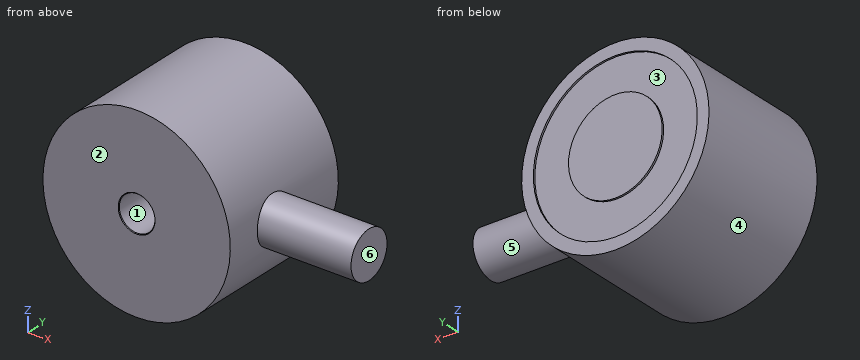
```python
from build123d import *

# Parameters (mm, degrees)
SKETCH1_R           = 12.7
BOSS_EXTRUDE1_DEPTH = 19.05
SKETCH2_W           = 4.7625
SKETCH2_H           = 0.254
SKETCH3_R           = 2.413
CUT_EXTRUDE1_DEPTH  = 9.525
BOSS_EXTRUDE2_START = 25.4
SKETCH7_R           = 3.175
BOSS_EXTRUDE2_DEPTH = 13.103277876


# Read off the part's stored shape, not the designer's step: Cut-Extrude2
with BuildPart() as part:
    # Sketch1 → Boss-Extrude1 (new body)
    with BuildSketch(Plane(origin=(0, 0, 0), x_dir=(1, 0, 0), z_dir=(0, 1, 0))):
        with Locations(Location((0, 0, 0), (0, 0, 90))):
            Circle(SKETCH1_R)
    extrude(amount=BOSS_EXTRUDE1_DEPTH)

    # Sketch2 → Cut-Revolve1 (revolve, cut)
    with BuildSketch(Plane.XY, mode=Mode.PRIVATE) as cut_revolve1_sk:
        with Locations((-8.73125, 18.923)):
            Rectangle(SKETCH2_W, SKETCH2_H)
    revolve(cut_revolve1_sk.sketch.rotate(Axis((0, 0, 0), (0, 1, 0)), 270), axis=Axis((0, 0, 0), (0, 1, 0)), mode=Mode.SUBTRACT)

    # Sketch3 → Cut-Extrude1 (cut)
    with BuildSketch(Plane.XZ):
        with Locations(Location((0, 0, 0), (0, 0, 270))):
            Circle(SKETCH3_R)
    extrude(amount=-CUT_EXTRUDE1_DEPTH, mode=Mode.SUBTRACT)

    # Cut-Extrude2 outline → Cut-Extrude2 (revolve, cut)
    with BuildSketch(Plane.XY):
        Polygon((2.498925958, 0), (2.413, 0.085925958), (2.413, 0), align=None)
    revolve(axis=Axis((0, 0, 0), (0, 1, 0)), mode=Mode.SUBTRACT)

    # Sketch7 → Boss-Extrude2 (add)
    with BuildSketch(Plane(origin=(0, 0, 0), x_dir=(0, 0, -1), z_dir=(1, 0, 0)).offset(BOSS_EXTRUDE2_START)):
        with Locations((0, 7.9375)):
            Circle(SKETCH7_R)
    extrude(amount=-BOSS_EXTRUDE2_DEPTH)


solid = part.part
```
Input: part model. Units: mm. Frame: model coordinates. Face numbers are marked on the shaded views. A direction names the side the tool comes from. Coordinates: 2 decimals unless noted, no trailing zeros. Loops run counter-clockwise (first coordinate to the right, second up) from the corner with the lowest first, then second, coordinate; pieces in that order, holes last.
Q1. Section C-C, the plane y = 5.5. Return the cut outline in (x, z).
Results are:
outline: (12.54, -2.03) - (25.4, -2.03) - (25.4, 2.03) - (12.54, 2.03) arc R12.7 ccw (long way) to start; hole circle Ø4.83 at (0, 0)
Q2. Mould query, pull axis X, two halves, no side actions, for the marked faces 3, 4, 5 and 6. Classes: +X half, -X half, draft (parallel to the pull), parting line (faces both ways), or undercut.
Results are:
face 3: undercut
face 4: parting line
face 5: draft
face 6: +X half
Q3. Set-up query: the marked faces 1 and 2. Return all of +Z, -Z, +X, -X, +Y, -Y with unobstructed straight access to the full face (end or side cutting, diameter ignored); none if empty.
Results are:
face 1: -Y
face 2: +Z, -Z, +X, -X, -Y
Q4. Line query: line 1 along X through (y, z) = (4.5, 0); line 2 along Y through (x, z) = (-1.5, -6.5); line 3 along X through (y, z) = (15.5, -0.5). Output: solid intervals per line, ascending.
Results are:
line 1: x = -12.7 to -2.41, 2.41 to 12.7
line 2: y = 0 to 18.8
line 3: x = -12.69 to 12.69
Q5. Section D-D, the plane x = -4. Return the cut outline in (y, z), and give its area (3 significant figures).
Results are:
outline: (0, -12.05) - (19.05, -12.05) - (19.05, -10.37) - (18.8, -10.37) - (18.8, -4.93) - (19.05, -4.93) - (19.05, 4.93) - (18.8, 4.93) - (18.8, 10.37) - (19.05, 10.37) - (19.05, 12.05) - (0, 12.05) - close
area: 456 mm2
Q6. Contact query for flat-ended pins moving along their axis: pin 1 (5 mm diameter, centred on x = 9, y = 7, fed in from +Z); pin 2 (2.5 mm diameter, centred on x = 0.5, z = 0.5, fed in from -Y) (3 decimals); pin 3 (2 mm diameter, centred on x = 15, y = 6, fed in from -Z). Output: stop coordinate, or through.
Results are:
pin 1: stops at z = 10.91
pin 2: stops at y = 9.525
pin 3: stops at z = -3.03
